from build123d import *

# Parameters (mm, degrees)
SKETCH_1_R      = 1.6
EXTRUDE_1_DEPTH = 3
EXTRUDE_START   = 3
EXTRUDE_3_DEPTH = 3


with BuildPart() as part:
    # 草图1 → 凸台-拉伸1 (new body)
    with BuildSketch(Plane(origin=(0, 0, 0), x_dir=(1, 0, 0), z_dir=(0, 1, 0))):
        with BuildLine():
            Line((-0.009028181, 21.389975432), (-0.009028181, -28.591736531))
            ThreePointArc((-0.009028181, -28.591736531), (-0.887707838, -30.713056875), (-3.009028181, -31.591736531))
            Line((-3.009028181, -31.591736531), (-77.021723127, -31.591736531))
            ThreePointArc((-77.021723127, -31.591736531), (-79.134066788, -30.716775138), (-80.009028181, -28.604431477))
            Line((-80.009028181, -28.604431477), (-80.009028181, 21.402670377))
            ThreePointArc((-80.009028181, 21.402670377), (-79.134066788, 23.515014039), (-77.021723127, 24.389975432))
            Line((-77.021723127, 24.389975432), (-3.009028181, 24.389975432))
            ThreePointArc((-3.009028181, 24.389975432), (-0.887707838, 23.511295776), (-0.009028181, 21.389975432))
        make_face()
        with Locations(Location((-76.52848462, 20.886724226, 0), (0, 0, 270))):
            Circle(SKETCH_1_R, mode=Mode.SUBTRACT)
        with Locations(Location((-18.52858622, 20.886597225, 0), (0, 0, 270))):
            Circle(SKETCH_1_R, mode=Mode.SUBTRACT)
        with Locations(Location((-18.52833222, -28.113656775, 0), (0, 0, 270))):
            Circle(SKETCH_1_R, mode=Mode.SUBTRACT)
        with Locations(Location((-76.52833222, -28.113529775, 0), (0, 0, 270))):
            Circle(SKETCH_1_R, mode=Mode.SUBTRACT)
        with BuildLine():
            Line((-70.770059731, 18.230282987), (-55.140568984, 18.230282987))
            ThreePointArc((-55.140568984, 18.230282987), (-54.292040846, 17.878811124), (-53.940568984, 17.030282987))
            Line((-53.940568984, 17.030282987), (-53.940568984, -23.088422311))
            ThreePointArc((-53.940568984, -23.088422311), (-54.292040846, -23.936950448), (-55.140568984, -24.288422311))
            Line((-55.140568984, -24.288422311), (-70.770059731, -24.288422311))
            ThreePointArc((-70.770059731, -24.288422311), (-71.618587868, -23.936950448), (-71.970059731, -23.088422311))
            Line((-71.970059731, -23.088422311), (-71.970059731, 17.030282987))
            ThreePointArc((-71.970059731, 17.030282987), (-71.618587868, 17.878811124), (-70.770059731, 18.230282987))
        make_face(mode=Mode.SUBTRACT)
    extrude(amount=EXTRUDE_1_DEPTH)

    # 草图3 → 凸台-拉伸3 (add)
    with BuildSketch(Plane.XZ.offset(EXTRUDE_START)):
        with BuildLine():
            Line((-15.227079657, 31.591736531), (-3.009028181, 31.591736531))
            ThreePointArc((-3.009028181, 31.591736531), (-0.887707838, 30.713056875), (-0.009028181, 28.591736531))
            Line((-0.009028181, 28.591736531), (-0.009028181, -21.389975432))
            ThreePointArc((-0.009028181, -21.389975432), (-0.887707838, -23.511295776), (-3.009028181, -24.389975432))
            Line((-3.009028181, -24.389975432), (-15.227079657, -24.389975432))
            Line((-15.227079657, -24.389975432), (-15.227079657, 31.591736531))
        make_face()
    extrude(amount=-EXTRUDE_3_DEPTH)


solid = part.part
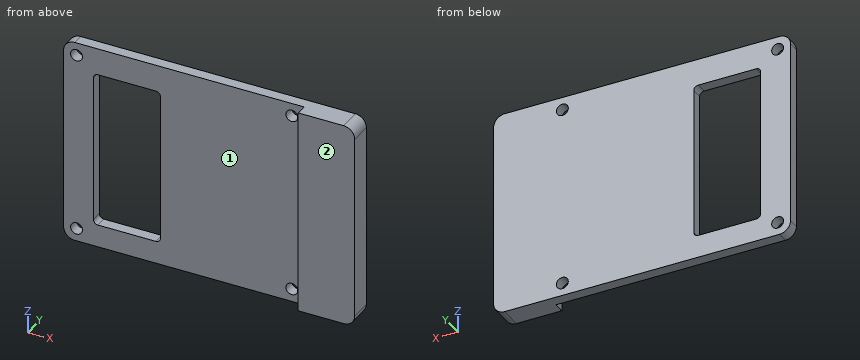
Geometry: final body of the model. Coordinates: model frame, mm. Face numbers are marked on the shaded views. A direction names the side the tool comes from. Coordinates: 2 decimals unless noted, no trailing zeros. Loops run counter-clockwise (first coordinate to the right, second up) from the corner with the lowest first, then second, coordinate; pieces in that order, holes last. Notation, with made-up numbers: M 67.25,48 L 77.25,48 A26 cw 77.25,79 Z; hole C 38,84 d8. An arc over 180 degrees is marked long. One line per item, written item: value. Start each with the question number.
1) Pin query (flat end, axial travel): P1, Ø2.5, axis at x = -76.53, z = 28.11, coming from the -Y side; P2, Ø5, axis at x = -28, z = -17, coming from the -Y side. Return the tip coordinate at first contact, or that it passes through.
2) Material intervals for L1, parallel to Z at x = -59.5, y = 1; L2, parallel to X at y = 0.7, z = -0.5; L3, parallel to Y at x = -53, z = -10, sorted ascending. Write a range as from..to.
3) Cut plane B-B (x = -69). Return loops of the section in (y, z), then the cut area to 3 significant figures.
4) Reachability of the marked faces 1 and 2 from +Z, -Z, +X, -X, +Y, -Y: full face, straight path, thin tool, end or side. Return the list, or none.
5) Cut plane D-D (y = 1.45). Return loops of the section in (x, z).
6) Cut plane A-A (z = 12). Return loops of the section in (x, y).
7) Cut plane C-C (y = -2.2). Return loops of the section in (x, z), then the cut area to 3 significant figures.
Evaluation:
1. P1: through
1. P2: y = 0
2. L1: -24.39..-18.23, 24.29..31.59
2. L2: -80.01..-71.97, -53.94..-0.01
2. L3: 0..3
3. outline: M 0,-24.39 L 3,-24.39 L 3,-18.23 L 0,-18.23 Z; M 0,24.29 L 3,24.29 L 3,31.59 L 0,31.59 Z
3. area: 40.4 mm^2
4. face 1: +Z, -Z, -X, -Y
4. face 2: +Z, -Z, +X, -X, -Y
5. outline: M -80.01,-21.4 A2.99 ccw -77.02,-24.39 L -3.01,-24.39 A3 ccw -0.01,-21.39 L -0.01,28.59 A3 ccw -3.01,31.59 L -77.02,31.59 A2.99 ccw -80.01,28.6 Z; hole C -76.53,-20.89 d3.2; hole C -76.53,28.11 d3.2; hole M -71.97,-17.03 A1.2 ccw -70.77,-18.23 L -55.14,-18.23 A1.2 ccw -53.94,-17.03 L -53.94,23.09 A1.2 ccw -55.14,24.29 L -70.77,24.29 A1.2 ccw -71.97,23.09 Z; hole C -18.53,-20.89 d3.2; hole C -18.53,28.11 d3.2
6. outline: M -80.01,0 L -71.97,0 L -71.97,3 L -80.01,3 Z; M -53.94,0 L -15.23,0 L -15.23,-3 L -0.01,-3 L -0.01,3 L -53.94,3 Z
7. outline: M -15.23,-24.39 L -3.01,-24.39 A3 ccw -0.01,-21.39 L -0.01,28.59 A3 ccw -3.01,31.59 L -15.23,31.59 Z
7. area: 848 mm^2
